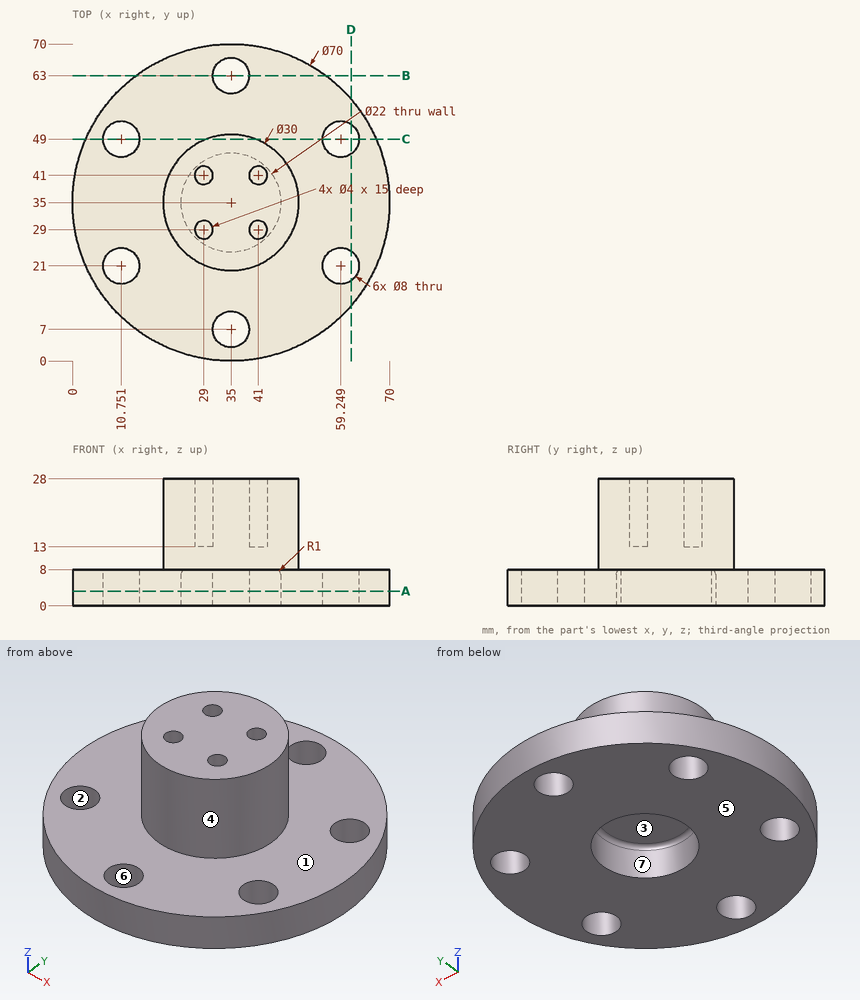
For this review, use the dimensioned drawing (mm, ordinates from the lowest corner) and the shaded views. A direction names the side the tool comes from. Give positions to 0.01 mm unless a question says otherwise; leave off trailing zeros. Loops run counter-clockwise (first coordinate to the right, second up) from the corner with the lowest first, then second, coordinate; pieces in that order, holes last. Notation, with made-up numbers: (66, 65.25) -> (103, 65.25) arc R24 cw to (103, 94.25) -> close; hole circle Ø11 at (-17.75, -38.5). An arc over 180 degrees is marked (long way). Use CSV: the item, a comma, the result in double quotes.
1. Consider section B-B, the plane y = 63. Write out the cut boundary in (x, z), then the cut area to 3 significant figures.
Result:
outline,"(14, 0) -> (31, 0) -> (31, 8) -> (14, 8) -> close; (39, 0) -> (56, 0) -> (56, 8) -> (39, 8) -> close"
area,"272 mm²"
2. Consider section C-C, the plane y = 49. Write out the cut boundary in (x, z) (1 decimal).
Result:
outline,"(2.9, 0) -> (6.8, 0) -> (6.8, 8) -> (2.9, 8) -> close; (14.8, 0) -> (55.2, 0) -> (55.2, 8) -> (40.4, 8) -> (40.4, 28) -> (29.6, 28) -> (29.6, 8) -> (14.8, 8) -> close; (63.2, 0) -> (67.1, 0) -> (67.1, 8) -> (63.2, 8) -> close"
3. To check wall thickness, follow probe 1 along Y at (x, z) = (35, 5.75); probe 2 along Y at (x, z) = (41, 21.75); probe 3 along Y at (x, z) = (40, 18). State the ranges of each line that lie inside material, in increasing order. Write a range as from..to.
Result:
probe 1,"y = 0..3, 11..24, 46..59, 67..70"
probe 2,"y = 21.25..27, 31..39, 43..48.75"
probe 3,"y = 20.86..27.27, 30.73..39.27, 42.73..49.14"
4. Machinability: for the marked faces 1, 2 and 3, which of the approach directions +Z, -Z, +X, -X, +Y, -Y give a long, thin tool a straight path to every point of the face, cutting with its end or side? Answer none if there is none.
Result:
face 1,"+Z"
face 2,"+Z, -Z"
face 3,"-Z"
5. For P1, Ø3, axis at x = 19.5, y = 20, coming from the +Z side; P2, Ø6, axis at y = 34, z = 24.5, coming from the +X side; P3, Ø1, axis at x = 18, y = 60.5, coming from the -Z side; P4, Ø5, axis at x = 40.5, y = 36, coming from the -Z side, all flat-tipped, find the tip position at first contact; note any pin that passes through.
Result:
P1,"stops at z = 8"
P2,"stops at x = 50"
P3,"stops at z = 0"
P4,"stops at z = 8"
6. Consider section A-A, the plane z = 3.25. Write out the cut boundary in (x, y).
Result:
outline,"circle Ø70 at (35, 35); hole circle Ø8 at (10.75, 21); hole circle Ø8 at (10.75, 49); hole circle Ø22 at (35, 35); hole circle Ø8 at (35, 7); hole circle Ø8 at (35, 63); hole circle Ø8 at (59.25, 21); hole circle Ø8 at (59.25, 49)"
7. The part is to be moulded in two halves that separate along X. For the marked faces 4, 5, 6 and 7, say which applies: +X half, -X half, draft (parallel to the pull), parting line (faces both ways), or undercut.
Result:
face 4,"parting line"
face 5,"draft"
face 6,"undercut"
face 7,"undercut"
8. Consider section D-D, the plane x = 61.5. Write out the cut boundary in (y, z), then the cut area to 3 significant figures.
Result:
outline,"(12.14, 0) -> (17.69, 0) -> (17.69, 8) -> (12.14, 8) -> close; (24.31, 0) -> (45.69, 0) -> (45.69, 8) -> (24.31, 8) -> close; (52.31, 0) -> (57.86, 0) -> (57.86, 8) -> (52.31, 8) -> close"
area,"260 mm²"
